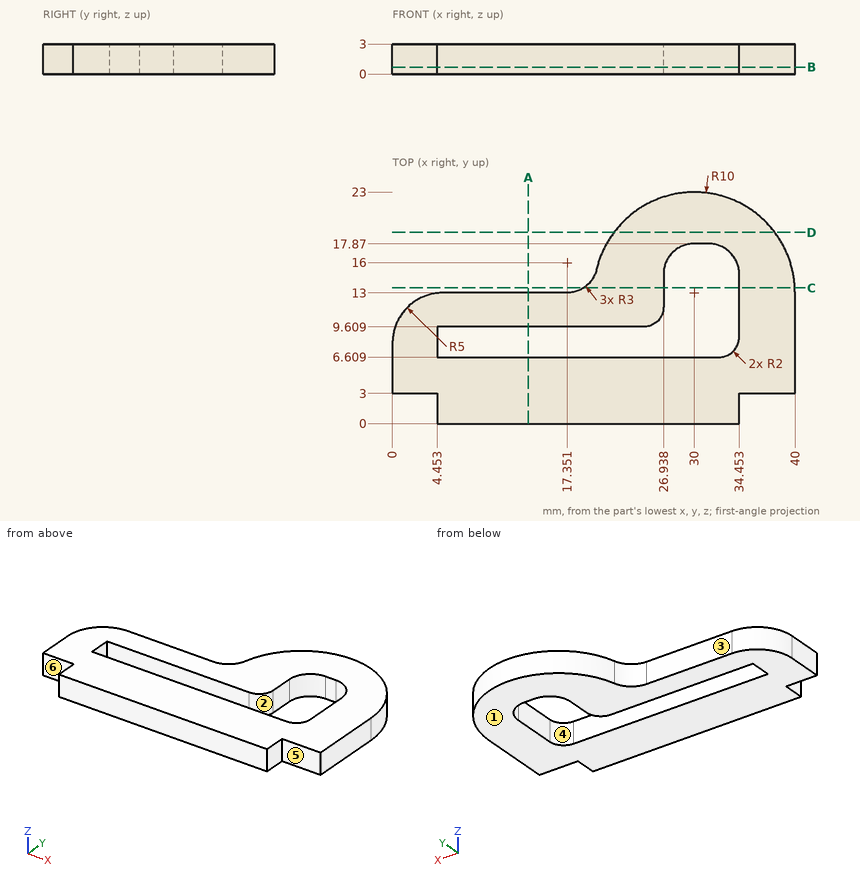
Can you work these out from the drawing? Everything is in mm from the part's minimum corner. A direction names the side the tool comes from. Round coordinates to 2 decimals unless told otherwise and drop trailing zeros. Loops run counter-clockwise (first coordinate to the right, second up) from the corner with the lowest first, then second, coordinate; pieces in that order, holes last. Notation, with made-up numbers: (44, 34) -> (79, 34) arc R14 ccw to (79, 61) -> close; hole circle Ø2 at (35, -35.75). An arc over 180 degrees is marked (long way). Use CSV: the item, a comma, the result in double quotes.
(1) If we mould it in two halves opening along Y, with no side actions, what happens to the marked faces 1, 2 and 3? For each: +Y half, -Y half, draft (parallel to the pull), parting line (faces both ways), or undercut.
Return value:
face 1,"draft"
face 2,"undercut"
face 3,"+Y half"
(2) Suppose I cut it at D-D on y = 19. Write out the boundary of the cut face in (x, z).
Return value:
outline,"(22, 0) -> (38, 0) -> (38, 3) -> (22, 3) -> close"
(3) If I drill on probe 1 along Y at (x, z) = (14.5, 0.8); probe 2 along X at (y, z) = (2.75, 1.9); probe 3 along Y at (x, z) = (32.5, 1.8), over which ranges is the centre line in solid material (lowest first)? Write a range as [from, to].
Return value:
probe 1,"y = [0, 6.61], [9.61, 13]"
probe 2,"x = [4.45, 34.45]"
probe 3,"y = [0, 6.61], [17.68, 22.68]"
(4) Will this pin go through, and if not, where does the flat tip stop? pin 1 Ø1.5 at (x, z) = (16.5, 2.5) entering from +Y.
Return value:
pin 1,"stops at y = 13"
(5) For the marked faces 4, 5 and 6, which set-ups out of +Z, -Z, +X, -X, +Y, -Y let a thin tool reach every point of the face, with its end or its side?
Return value:
face 4,"+Z, -Z"
face 5,"+Z, -Z, +X, -Y"
face 6,"+Z, -Z, -X, -Y"
(6) Suppose I cut it at B-B on z = 0.7. Write out the boundary of the cut face in (x, y), plus the area to 3 significant figures.
Return value:
outline,"(0, 3) -> (4.45, 3) -> (4.45, 0) -> (34.45, 0) -> (34.45, 3) -> (40, 3) -> (40, 13) arc R10 ccw to (20.27, 15.31) arc R3 cw to (17.35, 13) -> (5, 13) arc R5 ccw to (0, 8) -> close; hole (4.45, 6.61) -> (32.45, 6.61) arc R2 ccw to (34.45, 8.61) -> (34.45, 14.87) arc R3 ccw to (31.45, 17.87) -> (29.94, 17.87) arc R3 ccw to (26.94, 14.87) -> (26.94, 11.61) arc R2 cw to (24.94, 9.61) -> (4.45, 9.61) -> close"
area,"495 mm²"
(7) Suppose I cut it at A-A on x = 13.5. Write out the boundary of the cut face in (y, z).
Return value:
outline,"(0, 0) -> (6.61, 0) -> (6.61, 3) -> (0, 3) -> close; (9.61, 0) -> (13, 0) -> (13, 3) -> (9.61, 3) -> close"
(8) Suppose I cut it at C-C on y = 13.5. Write out the boundary of the cut face in (x, z), plus the area to 3 significant figures.
Return value:
outline,"(19.01, 0) -> (26.94, 0) -> (26.94, 3) -> (19.01, 3) -> close; (34.45, 0) -> (39.99, 0) -> (39.99, 3) -> (34.45, 3) -> close"
area,"40.4 mm²"
